For this review, take the finished solid that the model builds, in its own axes (mm). Face numbers are marked on the shaded views. Round coordinates to 2 decimals unless told otherwise and drop trailing zeros. Write each loop counter-clockwise with the first axis right and the second up, starting at its lowest first coordinate (ties: lowest second). Pieces come first, ordered by that corner, then holes. Notation, with made-up numbers: (59.5, 78.25) -> (88.5, 78.25) arc R20 cw to (88.5, 115.25) -> close; hole circle Ø5 at (4.25, 78.25). An arc over 180 degrees is marked (long way). Answer as CSV lines item,"result". Start each with the question number.
Item 1: For pin 1 Ø11.5 at (y, z) = (2.5, 23.5) entering from -X; pin 2 Ø24 at (x, y) = (-20.23, 0) entering from +Z, all flat-tipped, find the tip position at first contact; note any pin that passes through.
Item 2: Take a section at B-B on z = 29. Give the boundary of the cut face in (x, y).
Item 3: Wall thickness on probe 1 along Y at (x, z) = (0.45, 9); probe 2 along Y at (x, z) = (0.45, 29); probe 3 along Z at (x, y) = (-34, -16): over which ranges is each line inside the solid? List them lowest first. Write a range as from..to.
Item 4: Mouldability with a two-part tool opening along Z and no side actions: class the marked faces 1, 2 and 3 as +Z half, -Z half, draft (parallel to the pull), parting line (faces both ways), or undercut.
Item 5: Take a section at A-A on y = 15. Give the boundary of the cut face in (x, z).
Item 6: Take a section at D-D on x = -9. Give the boundary of the cut face in (y, z), then the cut area to 3 significant figures.
Item 7: Take a section at C-C on y = 0. Give the boundary of the cut face in (x, z), then the cut area to 3 significant figures.
```python
from build123d import *

# Parameters (mm, degrees)
SKETCH1_W               = 80
SKETCH1_H               = 40
BASE_FLANGE1_DEPTH      = 1
SKETCHED_START          = -20
SKETCHED_BEND1_DEPTH    = 40
SKETCHED_BEND1_2_DEPTH  = 40
FILLET1_R               = 2
SKETCH9_R               = 1.55
CUT_EXTRUDE1_DEPTH      = 60.687271317
CUT_EXTRUDE3_DEPTH      = 61.512940202
CUT_EXTRUDE3_DEPTH_BACK = 61.512940202
SKETCH10_R              = 7.5
CHAMFER1_SIZE           = 0.5


# Read off the part's stored shape, not the designer's step: Sketched Bend1
# Sheet-metal steps are written as plain solids
with BuildPart() as part:
    # Sketch1 → Base-Flange1 (new body)
    with BuildSketch(Plane.XY):
        Rectangle(SKETCH1_W, SKETCH1_H)
    extrude(amount=-BASE_FLANGE1_DEPTH)

    # Sketched Bend1 outline → Sketched Bend1 (cut)
    with BuildSketch(Plane(origin=(0, 0, 0), x_dir=(1, 0, 0), z_dir=(0, 1, 0)).offset(SKETCHED_START)):
        with BuildLine():
            ThreePointArc((-0.971223369, 1), (-0.039397205, 0.728828115), (0.601417721, 0))
            Line((0.601417721, 0), (40, 0))
            Line((40, 0), (40, 1))
            Line((40, 1), (-0.971223369, 1))
        make_face()
    extrude(amount=SKETCHED_BEND1_DEPTH, mode=Mode.SUBTRACT)

    # Sketched Bend1 2 outline → Sketched Bend1 2 (add)
    with BuildSketch(Plane(origin=(0, 0, 0), x_dir=(1, 0, 0), z_dir=(0, 1, 0)).offset(SKETCHED_START)):
        with BuildLine():
            Line((-0.234623369, -0.7366), (-0.234623369, -39.765376631))
            Line((-0.234623369, -39.765376631), (0.765376631, -39.765376631))
            Line((0.765376631, -39.765376631), (0.765376631, -0.7366))
            ThreePointArc((0.765376631, -0.7366), (0.723891388, -0.359286442), (0.601417721, 0))
            Line((0.601417721, 0), (-0.971223369, 0))
            ThreePointArc((-0.971223369, 0), (-0.450368514, -0.215745145), (-0.234623369, -0.7366))
        make_face()
    extrude(amount=SKETCHED_BEND1_2_DEPTH)

    # Fillet1
    fillet1_edges = [part.edges().sort_by_distance(p)[0] for p in [
        (-40, -20, -0.5),
        (-40, 20, -0.5),
        (0.265376631, -20, 39.765376631),
        (0.265376631, 20, 39.765376631),
    ]]
    fillet(fillet1_edges, radius=FILLET1_R)

    # Sketch9 → Cut-Extrude1 (cut, through all)
    with BuildSketch(Plane.ZY.offset(0.234623369)):
        with Locations((9, 15)):
            Circle(SKETCH9_R)
        with Locations((29, 10)):
            Circle(SKETCH9_R)
        with Locations(Location((29, -10, 0), (0, 0, 180))):
            Circle(SKETCH9_R)
        with Locations(Location((9, -15, 0), (0, 0, 180))):
            Circle(SKETCH9_R)
    extrude(amount=-CUT_EXTRUDE1_DEPTH, mode=Mode.SUBTRACT)

    # Sketch10 → Cut-Extrude3 (cut, two sides: drawn at the far end of the back side and taken through both)
    with BuildSketch(Plane(origin=(0, 0, -1), x_dir=(-1, 0, 0), z_dir=(0, 0, -1)).offset(-CUT_EXTRUDE3_DEPTH_BACK)):
        with Locations((20.234623369, 0)):
            Circle(SKETCH10_R)
    extrude(amount=CUT_EXTRUDE3_DEPTH + CUT_EXTRUDE3_DEPTH_BACK, mode=Mode.SUBTRACT)

    # Chamfer1
    chamfer1_edges = [part.edges().sort_by_distance(p)[0] for p in [
        (-0.234623369, 15, 7.45),
        (-0.234623369, 10, 27.45),
        (-0.234623369, -10, 30.55),
        (-0.234623369, -15, 10.55),
    ]]
    chamfer(chamfer1_edges, length=CHAMFER1_SIZE)


solid = part.part
```
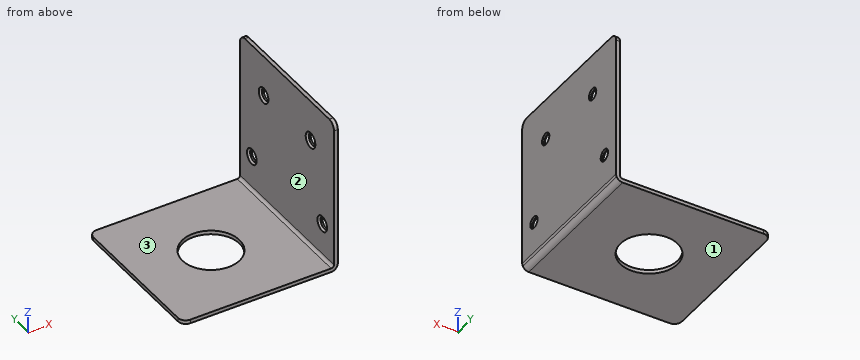
Output values:
1,pin 1,"stops at x = -0.23"
1,pin 2,"stops at z = 0"
2,outline,"(-0.23, -20) -> (0.77, -20) -> (0.77, -11.55) -> (0.27, -11.55) -> (-0.23, -12.05) -> close; (-0.23, -7.95) -> (0.27, -8.45) -> (0.77, -8.45) -> (0.77, 8.45) -> (0.27, 8.45) -> (-0.23, 7.95) -> close; (-0.23, 12.05) -> (0.27, 11.55) -> (0.77, 11.55) -> (0.77, 20) -> (-0.23, 20) -> close"
3,probe 1,"y = -20..-16.55, -13.45..13.45, 16.55..20"
3,probe 2,"y = -20..-11.55, -8.45..8.45, 11.55..20"
3,probe 3,"z = -1..0"
4,face 1,"-Z half"
4,face 2,"draft"
4,face 3,"+Z half"
5,outline,"(-40, -1) -> (-0.97, -1) arc R1.74 ccw to (0.77, 0.74) -> (0.77, 7.45) -> (0.27, 7.45) -> (-0.23, 6.95) -> (-0.23, 0.74) arc R0.74 cw to (-0.97, 0) -> (-40, 0) -> close; (-0.23, 11.05) -> (0.27, 10.55) -> (0.77, 10.55) -> (0.77, 39.77) -> (-0.23, 39.77) -> close"
6,outline,"(-20, -1) -> (20, -1) -> (20, 0) -> (-20, 0) -> close"
6,area,"40.0 mm^2"
7,outline,"(-40, -1) -> (-27.73, -1) -> (-27.73, 0) -> (-40, 0) -> close; (-12.73, -1) -> (-0.97, -1) arc R1.74 ccw to (0.77, 0.74) -> (0.77, 39.77) -> (-0.23, 39.77) -> (-0.23, 0.74) arc R0.74 cw to (-0.97, 0) -> (-12.73, 0) -> close"
7,area,"65.0 mm^2"
